from build123d import *

# Parameters (mm, degrees)
F0_W     = 12.7
F0_H     = 508
F1_DEPTH = 12.5222
F2_R     = 2.452841


with BuildPart() as f1:
    # F0 (on Top) → F1 (new body)
    with BuildSketch(Plane.XY):
        with BuildLine():
            Line((-74.624596, 605.821555), (-557.224596, 605.821555))
            Line((-557.224596, 605.821555), (-557.224596, 555.021555))
            Line((-557.224596, 555.021555), (-557.224596, 47.021555))
            Line((-557.224596, 47.021555), (-557.224596, -3.778445))
            Line((-557.224596, -3.778445), (-74.624596, -3.778445))
            ThreePointArc((-74.624596, -3.778445), (15.177965, 33.418993), (52.375404, 123.221555))
            Line((52.375404, 123.221555), (52.375404, 478.821555))
            ThreePointArc((52.375404, 478.821555), (15.177965, 568.624116), (-74.624596, 605.821555))
        make_face()
        with Locations((-563.574596, 301.021555)):
            Rectangle(F0_W, F0_H)
    extrude(amount=F1_DEPTH)

    # F2
    f2_edges = [f1.edges().sort_by_distance(p)[0] for p in [
        (52.375404, 301.021555, 12.5222),
        (15.177965, 568.624116, 12.5222),
        (-315.924596, 605.821555, 12.5222),
        (-557.224596, 580.421555, 12.5222),
        (-563.574596, 555.021555, 12.5222),
        (-569.924596, 301.021555, 12.5222),
        (-563.574596, 47.021555, 12.5222),
        (-557.224596, 21.621555, 12.5222),
        (-315.924596, -3.778445, 12.5222),
        (15.177965, 33.418993, 12.5222),
    ]]
    fillet(f2_edges, radius=F2_R)


solid = f1.part
The listing builds one solid part. Answer for the finished solid, in the listing's coordinates (mm). Give positions to 0.01 mm unless a question says otherwise; leave off trailing zeros. Write each loop counter-clockwise with the first axis right and the second up, starting at its lowest first coordinate (ties: lowest second). Pieces come first, ordered by that corner, then holes.
Item 1: Section A-A, the plane z = 6.25 is taken. Write down the section's boundary in (x, y).
Item 2: Flat-ended cylindrical pins translate along their axes: P1, Ø1, axis at x = -23, z = 5.5, coming from the +Y side; P2, Ø4, axis at y = 499, z = 3, coming from the +X side; P3, Ø5, axis at x = -561, z = 7, coming from the -Y side. Find the tip coordinate at first contact, or state that the pin passes through.
Item 3: Find the intervals of material crossed by line 1 along X through (y, z) = (481, 6.25); line 2 along X through (y, z) = (497.5, 8); line 3 along Y through (x, z) = (0, 7), in increasing order.
Completed:
1. outline: (-569.92, 47.02) - (-557.22, 47.02) - (-557.22, -3.78) - (-74.62, -3.78) arc R127 ccw to (52.38, 123.22) - (52.38, 478.82) arc R127 ccw to (-74.62, 605.82) - (-557.22, 605.82) - (-557.22, 555.02) - (-569.92, 555.02) - close
2. P1: stops at y = 595.08
2. P2: stops at x = 51.07
2. P3: stops at y = 47.02
3. line 1: x = -569.92 to 52.36
3. line 2: x = -569.92 to 50.99
3. line 3: y = 20.46 to 581.58
